Part model, mm, in its own coordinate system. Round coordinates to 2 decimals unless told otherwise and drop trailing zeros. Loops run counter-clockwise (first coordinate to the right, second up) from the corner with the lowest first, then second, coordinate; pieces in that order, holes last. Notation, with made-up numbers: (-8.5, 1.25) -> (-2.5, 1.25) arc R21 ccw to (-2.5, 9.25) -> close; hole circle Ø11 at (87.25, 81.25). An arc over 180 degrees is marked (long way). Answer as a JSON object with one key per item and string values. Group by question number.
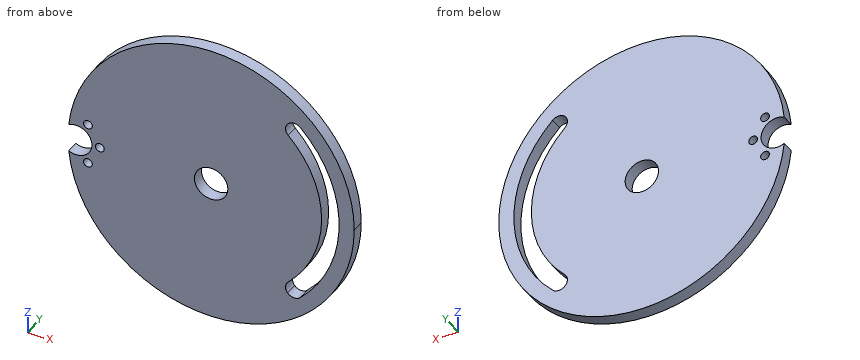
Solid Edge part; units mm, degrees
sketch "Sketch1" plane through (0, 0, 0) normal (0, -1, 0) x (1, 0, 0)
  circle A0 centre (0, 0) radius 90
extrude "Protrusion1" add sketch "Sketch1" along normal mid plane 8
sketch "Sketch2" plane through (0, -4, 0) normal (0, -1, 0) x (1, 0, 0)
  circle A0 centre (0, 0) radius 10.5
  circle A1 centre (-85, 0) radius 10
extrude "ExtrudedCutout_1" cut sketch "Sketch2" along normal mid plane 282.4978
extrude "ExtrudedCutout_2" [suppressed]
sketch "Sketch3" plane through (0, 4, 0) normal (0, 1, 0) x (-1, 0, 0)
  arc A0 (-44.6737, 53.2401) -> (-44.6737, -53.2401) centre (0, 0) ccw
  line L0 (-44.6737, -53.2401) -> (-51.7444, -61.6666)
  arc A1 (-51.7444, 61.6666) -> (-51.7444, -61.6666) centre (0, 0) ccw
  line L1 (-44.6737, 53.2401) -> (-51.7444, 61.6666)
extrude "ExtrudedCutout_3" cut sketch "Sketch3" against normal blind 80.1209
fillet "Round_2" radius 5.5 4 edges at (51.7444, 0, 61.6666) (44.6737, 0, 53.2401) (44.6737, 0, -53.2401) (51.7444, 0, -61.6666)
sketch "Sketch4" plane through (0.2206, 4, 0) normal (0, 1, 0) x (0, 0, 1)
  circle A0 centre (-12.9904, -77.7206) radius 2.75
  circle A1 centre (0, -70.2206) radius 2.75
  circle A2 centre (12.9904, -77.7206) radius 2.75
extrude "ExtrudedCutout_4" cut sketch "Sketch4" against normal blind 34.5178
properties material "PVC"
Item 1: Drop flat-ended pins along their axis: pin 1 Ø7 at (x, z) = (-70, 0) entering from -Y; pin 2 Ø1 at (y, z) = (0.5, -30) entering from +X. Give the stop position or say it passes through.
Item 2: Band-saw the part on B-B, the plane z = -30. List the corners of the cut face in (x, y), plus the area to 3 significant figures.
Item 3: Band-saw the part on D-D, the plane x = -77.5. List the corners of the cut face in (y, z).
Item 4: Band-saw the part on C-C, the plane y = 2.5. Count the separate pieces of the cut face and the enclosed holes in it, plus the area to 3 significant figures.
Item 5: Band-saw the part on A-A, the plane x = 0. List the corners of the cut face in (y, z), plus the area to 3 significant figures.
Item 6: Drill centre lines: line 1 (X direction, y = -0.25, z = 15); line 2 (X direction, y = 1.75, z = -11.5); line 3 (Z direction, x = 61, y = -0.25). Where is each one in solid material? Low to high.
Entries:
{
 "1": {"pin 1": "y = -4", "pin 2": "x = 85.03"},
 "2": {"outline": "(-84.85, -4) -> (62.69, -4) -> (62.69, 4) -> (-84.85, 4) -> close; (74.7, -4) -> (84.85, -4) -> (84.85, 4) -> (74.7, 4) -> close", "area": "1,260 mm²"},
 "3": {"outline": "(-4, -45.76) -> (4, -45.76) -> (4, -15.74) -> (-4, -15.74) -> close; (-4, -10.24) -> (4, -10.24) -> (4, -6.61) -> (-4, -6.61) -> close; (-4, 6.61) -> (4, 6.61) -> (4, 10.24) -> (-4, 10.24) -> close; (-4, 15.74) -> (4, 15.74) -> (4, 45.76) -> (-4, 45.76) -> close"},
 "4": {"separate pieces": "1", "enclosed holes": "5", "area": "23,400 mm²"},
 "5": {"outline": "(-4, -90) -> (4, -90) -> (4, -10.5) -> (-4, -10.5) -> close; (-4, 10.5) -> (4, 10.5) -> (4, 90) -> (-4, 90) -> close", "area": "1,270 mm²"},
 "6": {"line 1": "-88.74 to -79.38, -75.62 to 67.86, 79.09 to 88.74", "line 2": "-89.26 to -79.81, -75.19 to 68.54, 79.67 to 89.26", "line 3": "-66.17 to -52.53, -33.31 to 33.31, 52.53 to 66.17"}
}
